Can you work these out from the model? Positions are in its coordinate system, mm. Give positions to 0.01 mm unless a question says otherwise; leave off trailing zeros. Loops run counter-clockwise (first coordinate to the right, second up) from the corner with the lowest first, then second, coordinate; pieces in that order, holes last. Notation, with made-up numbers: M 47.5,23.25 L 104.5,23.25 A8 cw 104.5,37.25 Z; hole C 44,-22.75 d10. An arc over 180 degrees is marked long. Use CSV: the item, a comma, the result in double quotes.
from build123d import *

# Parameters (mm, degrees)
SKETCH2_R = 7.5


with BuildPart() as part:
    # Sweep1: sweep along a path in Sketch1
    with BuildLine(Plane(origin=(0, 0, 0), x_dir=(1, 0, 0), z_dir=(0, 1, 0))) as sweep1_path:
        Line((63.33532453, 12.5), (42.492979812, 48.6))
        ThreePointArc((42.492979812, 48.6), (33.342344718, 57.750635095), (20.842344718, 61.1))
        Line((20.842344718, 61.1), (-20.842344718, 61.1))
        ThreePointArc((-20.842344718, 61.1), (-33.342344718, 57.750635095), (-42.492979812, 48.6))
        Line((-42.492979812, 48.6), (-63.33532453, 12.5))
        ThreePointArc((-63.33532453, 12.5), (-66.684689435, 0), (-63.33532453, -12.5))
        Line((-63.33532453, -12.5), (-42.492979812, -48.6))
        ThreePointArc((-42.492979812, -48.6), (-33.342344718, -57.750635095), (-20.842344718, -61.1))
        Line((-20.842344718, -61.1), (20.842344718, -61.1))
        ThreePointArc((20.842344718, -61.1), (33.342344718, -57.750635095), (42.492979812, -48.6))
        Line((42.492979812, -48.6), (63.33532453, -12.5))
        ThreePointArc((63.33532453, -12.5), (66.684689435, 0), (63.33532453, 12.5))
    # Sketch2 → Sweep1 (sweep)
    with BuildSketch(Plane(origin=(0, 0, 0), x_dir=(0, 0, -1), z_dir=(1, 0, 0))):
        with Locations((68.6, 0)):
            Circle(SKETCH2_R)
    sweep(path=sweep1_path.line)


solid = part.part
Q1. Please list where these lines run through material, in increasing order: L1, parallel to X at y = 1.5, z = -9.5; L2, parallel to Z at x = -26, y = 4.75; L3, parallel to X at y = -1.75, z = 20. Write a range as from..to.
Model answer:
L1,"-80.38..-64.97, 64.97..80.38"
L2,"-74.06..-62.29, 62.29..74.06"
L3,"-76.09..-59.24, 59.24..76.09"
Q2. I'm going to push flat-ended pins straight in: P1, Ø5, axis at x = 21.5, y = 2.5, coming from the -Z side; P2, Ø8, axis at x = -34, y = -1.5, coming from the -Z side; P3, Ø1.5, axis at x = -43.5, y = 3, coming from the +Z side; P4, Ø6, axis at y = -5.5, z = -14.5, coming from the -X side. Where does each tip first touch, or does it pass through?
Model answer:
P1,"z = -76.1"
P2,"z = -74.99"
P3,"z = 68.93"
P4,"x = -78.91"
Q3. If we mould it in two halves opening along X, with no side actions, what happens to faces 1 (the cylindrical face through (-0.292, -2.253, -75.754)), 2 (the cylindrical face through (65.46, -2.25, -38.13))? For each: released by +X, released by -X, zero draft, split by the parting line, or undercut.
Model answer:
face 1,"undercut"
face 2,"undercut"
Q4. I want a section at B-B, the plane x = 6. Please give me the cut outline in (y, z), then the cut area to 3 significant figures.
Model answer:
outline,"C 0,-68.6 d15; C 0,68.6 d15"
area,"353 mm2"
Q5. I want a section at A-A, the plane y = 0. Please give me the cut outline in (x, z).
Model answer:
outline,"M -76.33,-20 L -55.48,-56.1 A40 ccw -20.84,-76.1 L 20.84,-76.1 A40 ccw 55.48,-56.1 L 76.33,-20 A40 ccw 76.33,20 L 55.48,56.1 A40 ccw 20.84,76.1 L -20.84,76.1 A40 ccw -55.48,56.1 L -76.33,20 A40 ccw Z; hole M -63.34,-12.5 L -42.49,-48.6 A25 ccw -20.84,-61.1 L 20.84,-61.1 A25 ccw 42.49,-48.6 L 63.34,-12.5 A25 ccw 63.34,12.5 L 42.49,48.6 A25 ccw 20.84,61.1 L -20.84,61.1 A25 ccw -42.49,48.6 L -63.34,12.5 A25 ccw Z"
